Here's how the part is built. I have some questions about the finished solid (model axes, mm). A direction names the side the tool comes from. Round coordinates to 2 decimals unless told otherwise and drop trailing zeros. Write each loop counter-clockwise with the first axis right and the second up, starting at its lowest first coordinate (ties: lowest second). Pieces come first, ordered by that corner, then holes. Notation, with made-up numbers: (58.25, 64.5) -> (86.25, 64.5) arc R19 cw to (86.25, 97.5) -> close; hole circle Ø10 at (20.5, 10.25). An arc over 180 degrees is marked (long way). Put each result on its own line as item: value. Start each with the question number.
1. Which directions (+Z, -Z, +X, -X, +Y, -Y) give clear straight access to the entire face, cutting with the end or side of a thin tool? Please do faces 1 (the face through (12, -49, 0)), 2 (the face through (-12.465, -56.133, 0.493)).
2. Suppose I cut it at D-D (x = 60). Please give me the cut outline in (y, z).
3. We'd pull the mould along Y, two halves only. Please class faces 3 (the face through (-48, 17, 3)), 4 (the face through (47, -30, 1)), 5 (the face through (-55.55, -42.594, 1.479)): +Y half, -Y half, draft (parallel to the pull), parting line (faces both ways), or undercut.
4. I need wall thicknesses on probe 1 along Y at (x, z) = (0, 0.4); probe 2 along X at (y, z) = (44, 0.9); probe 3 along X at (y, z) = (28, 0.6). Which ranges of each line are inside material? Lowest first, please. Write a range as from..to.
5. Suppose I cut it at A-A (x = 0). Please give me the cut outline in (y, z).
6. Suppose I cut it at C-C (z = 0.45). Please give me the cut outline in (x, y).
```python
from build123d import *

# Parameters (mm, degrees)
SKETCH_R             = 70
PAD_DEPTH            = 3
SKETCH001_R          = 57.5
POCKET_DEPTH         = 1
SKETCH002_R          = 55
PAD001_DEPTH         = 3
SKETCH003_R          = 50
POCKET001_DEPTH      = 0.001
POCKET001_DEPTH_BACK = -3.001


with BuildPart() as part:
    # Sketch → Pad (new body)
    with BuildSketch(Plane.XY):
        Circle(SKETCH_R)
    extrude(amount=PAD_DEPTH)

    # Sketch001 → Pocket (cut)
    with BuildSketch(Plane.XY):
        Circle(SKETCH001_R)
    extrude(amount=POCKET_DEPTH, mode=Mode.SUBTRACT)

    # Sketch002 → Pad001 (join)
    with BuildSketch(Plane.XY):
        Circle(SKETCH002_R)
    extrude(amount=PAD001_DEPTH)

    # Sketch003 → Pocket001 (cut, two sides)
    with BuildSketch(Plane.XY) as pocket001_sk:
        Circle(SKETCH003_R)
    extrude(amount=-POCKET001_DEPTH, mode=Mode.SUBTRACT)
    extrude(pocket001_sk.sketch, amount=-POCKET001_DEPTH_BACK, mode=Mode.SUBTRACT)


solid = part.part
```
Verdict:
1. face 1: -Z, +X, -X, +Y, -Y
1. face 2: -Z
2. outline: (-36.06, 0) -> (36.06, 0) -> (36.06, 3) -> (-36.06, 3) -> close
3. face 3: draft
3. face 4: undercut
3. face 5: parting line
4. probe 1: y = -70..-57.5, -55..-50, 50..55, 57.5..70
4. probe 2: x = -54.44..-37.02, -33..-23.75, 23.75..33, 37.02..54.44
4. probe 3: x = -64.16..-50.22, -47.34..-41.42, 41.42..47.34, 50.22..64.16
5. outline: (-70, 0) -> (-57.5, 0) -> (-57.5, 1) -> (-55, 1) -> (-55, 0) -> (-50, 0) -> (-50, 3) -> (-70, 3) -> close; (50, 0) -> (55, 0) -> (55, 1) -> (57.5, 1) -> (57.5, 0) -> (70, 0) -> (70, 3) -> (50, 3) -> close
6. outline: circle Ø140 at (0, 0); circle Ø110 at (0, 0); hole circle Ø115 at (0, 0); hole circle Ø100 at (0, 0)
